```python
from build123d import *

# Parameters (mm, degrees)
BOSS_EXTRUDE1_DEPTH = 5
SKETCH2_W           = 10
SKETCH2_H           = 8
BOSS_EXTRUDE2_DEPTH = 5
SKETCH3_R           = 1.5
CUT_EXTRUDE1_DEPTH  = 8


with BuildPart() as part:
    # Sketch1 → Boss-Extrude1 (new body)
    with BuildSketch(Plane(origin=(0, 0, 0), x_dir=(1, 0, 0), z_dir=(0, 1, 0))):
        with BuildLine():
            Line((10, -4), (-10, -4))
            ThreePointArc((-10, -4), (-14, 0), (-10, 4))
            Line((-10, 4), (10, 4))
            ThreePointArc((10, 4), (14, 0), (10, -4))
        make_face()
    extrude(amount=BOSS_EXTRUDE1_DEPTH)

    # Sketch2 → Boss-Extrude2 (add)
    with BuildSketch(Plane(origin=(0, 5, 0), x_dir=(1, 0, 0), z_dir=(0, 1, 0))):
        Rectangle(SKETCH2_W, SKETCH2_H)
    extrude(amount=BOSS_EXTRUDE2_DEPTH)

    # Sketch3 → Cut-Extrude1 (cut)
    with BuildSketch(Plane(origin=(0, 10, 0), x_dir=(1, 0, 0), z_dir=(0, 1, 0))):
        with Locations(Location((0, 0, 0), (0, 0, 270))):  # turned: the seam where the file's is
            Circle(SKETCH3_R)
    extrude(amount=-CUT_EXTRUDE1_DEPTH, mode=Mode.SUBTRACT)


solid = part.part
```
Could you check a few things on this model? Use its own coordinates, in mm. A direction names the side the tool comes from. Give positions to 0.01 mm unless a question says otherwise; leave off trailing zeros. Loops run counter-clockwise (first coordinate to the right, second up) from the corner with the lowest first, then second, coordinate; pieces in that order, holes last. Notation, with made-up numbers: (13.5, -1.75) - (38.5, -1.75) arc R30 ccw to (38.5, 20.25) - close; hole circle Ø8 at (-9, 22.5). An arc over 180 degrees is marked (long way). Answer in a Markdown table with one row per item. Add a question column.
Q1. We'd pull the mould along X, two halves only. Please class faces 1 (the face through (0.45, 6.06, 1.43)), 2 (the face through (0, 2, 0)), 3 (the face through (-14, 2, 0)), 4 (the face through (10, 5, 0)): +X half, -X half, draft (parallel to the pull), parting line (faces both ways), or undercut.
Q2. If we section it at C-C (z = 0): List the corners of the cut face in (x, y) for me.
Q3. For pin 1 (1.5 mm diameter, centred on y = 7.5, z = -1.5, fed in from +X); pin 2 (4 mm diameter, centred on y = 7.5, z = 2, fed in from -X), each with a flat end and sliding along its axis, tell me the tip position at first contact or that it passes through.
Q4. If we section it at D-D (y = 5.25): List the corners of the cut face in (x, z) for me, plus the area to 3 significant figures.
Q5. If we section it at B-B (y = 3.25): List the corners of the cut face in (x, z) for me.
Q6. Which directions (+Z, -Z, +X, -X, +Y, -Y) give clear straight access to the entire face, cutting with the end or side of a thin tool? Please do faces 5 (the face through (0, 4, -4)), 6 (the face through (5, 7, 0)), 7 (the face through (-9, 5, 0)).
Q7. If we section it at A-A (x = 0): List the corners of the cut face in (y, z) for me.
Q8. Please list where these lines run through material, in increasing order: L1, parallel to X at y = 8, z = 0; L2, parallel to Y at x = -10.75, z = 2.75; L3, parallel to X at y = 4, z = 0. Write a range as from..to.
The answers:
| question | item | result |
|---|---|---|
| 1 | face 1 | undercut |
| 1 | face 2 | undercut |
| 1 | face 3 | -X half |
| 1 | face 4 | draft |
| 2 | outline | (-14, 0) - (14, 0) - (14, 5) - (5, 5) - (5, 10) - (1.5, 10) - (1.5, 2) - (-1.5, 2) - (-1.5, 10) - (-5, 10) - (-5, 5) - (-14, 5) - close |
| 3 | pin 1 | stops at x = 5 |
| 3 | pin 2 | stops at x = -5 |
| 4 | outline | (-5, -4) - (5, -4) - (5, 4) - (-5, 4) - close; hole circle Ø3 at (0, 0) |
| 4 | area | 72.9 mm^2 |
| 5 | outline | (-10, -4) - (10, -4) arc R4 ccw to (10, 4) - (-10, 4) arc R4 ccw to start; hole circle Ø3 at (0, 0) |
| 6 | face 5 | -Z, +X, -X, +Y, -Y |
| 6 | face 6 | +Z, -Z, +X, +Y |
| 6 | face 7 | +Z, -Z, -X, +Y |
| 7 | outline | (0, -4) - (10, -4) - (10, -1.5) - (2, -1.5) - (2, 1.5) - (10, 1.5) - (10, 4) - (0, 4) - close |
| 8 | L1 | x = -5..-1.5, 1.5..5 |
| 8 | L2 | y = 0..5 |
| 8 | L3 | x = -14..-1.5, 1.5..14 |
